Build history of the part. All positions in model axes, mm. Face numbers are marked on the shaded views. Round coordinates to 2 decimals unless told otherwise and drop trailing zeros. Write each loop counter-clockwise with the first axis right and the second up, starting at its lowest first coordinate (ties: lowest second). Pieces come first, ordered by that corner, then holes.
1) Saw through at A-A (y = -12.5). Write the cut outline in (x, z), plus the area to 3 significant figures.
2) Flat gauge pin, fed straight in: pin 1 (3 mm diameter, centred on x = -11.5, y = 16, fed in from -Z). Where does the tip first touch, or does it go through?
3) Pull direction X, two halves, no side cores. Call the marked faces 1, 2 and 3: +X half, -X half, draft (parallel to the pull), parting line (faces both ways), or undercut.
4) Wall check: probe 1 along X at (y, z) = (-30, 13); probe 2 along X at (y, z) = (-26.5, 6.5); probe 3 along Z at (x, y) = (3, -33). Give the ranges that are in metal, low to high.
5) Saw through at B-B (x = 0). Write the cut outline in (y, z), plus the area to 3 significant figures.
from build123d import *

# Parameters (mm, degrees)
SKETCH_1_W          = 100
SKETCH_1_H          = 100
EXTRUDE_1_DEPTH     = 100
SKETCH_2_R          = 20
CUT_EXTRUDE_1_DEPTH = 151


with BuildPart() as part:
    # 草图1 → 凸台-拉伸1 (new body)
    with BuildSketch(Plane.XY):
        Rectangle(SKETCH_1_W, SKETCH_1_H)
    extrude(amount=EXTRUDE_1_DEPTH)

    # 草图2 → 切除-拉伸1 (cut, through all)
    with BuildSketch(Plane(origin=(0, 50, 0), x_dir=(1, 0, 0), z_dir=(0, 1, 0))):
        Circle(SKETCH_2_R)
    extrude(amount=-CUT_EXTRUDE_1_DEPTH, mode=Mode.SUBTRACT)


solid = part.part
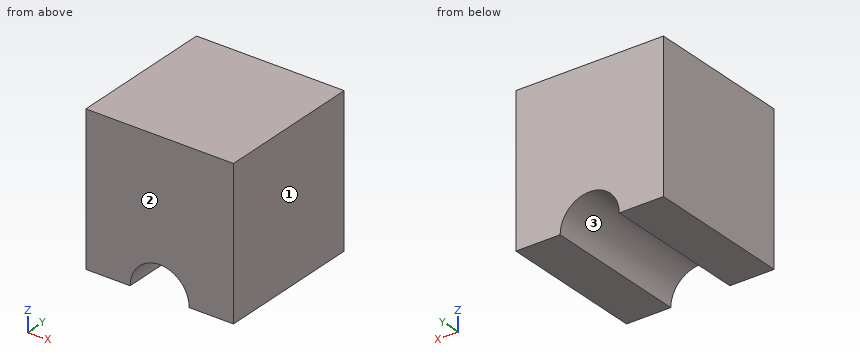
Evaluation:
1. outline: (-50, 0) - (-20, 0) arc R20 cw to (20, 0) - (50, 0) - (50, 100) - (-50, 100) - close
1. area: 9,370 mm2
2. pin 1: stops at z = 15.2
3. face 1: +X half
3. face 2: draft
3. face 3: undercut
4. probe 1: x = -50 to -15.2, 15.2 to 50
4. probe 2: x = -50 to -18.91, 18.91 to 50
4. probe 3: z = 19.77 to 100
5. outline: (-50, 20) - (50, 20) - (50, 100) - (-50, 100) - close
5. area: 8,000 mm2
